For this review, take the finished solid that the model builds, in its own axes (mm). Give positions to 0.01 mm unless a question says otherwise; leave off trailing zeros. Write each loop counter-clockwise with the first axis right and the second up, starting at its lowest first coordinate (ties: lowest second). Pieces come first, ordered by that corner, then holes. Notation, with made-up numbers: (-12, 33.25) -> (44, 33.25) arc R20 ccw to (44, 38.25) -> close; hole circle Ø8 at (79.5, 87). An arc over 180 degrees is marked (long way). Return JSON: item names as keys, results as strings.
from build123d import *

# Parameters (mm, degrees)
F0_R     = 2.75
F1_DEPTH = 6


with BuildPart() as f1:
    # F0 (on Top) → F1 (new body)
    with BuildSketch(Plane.XY):
        with BuildLine():
            Line((6.000003, -2.478286), (-4.999997, -2.478286))
            Line((-4.999997, -2.478286), (-4.999997, -8.478286))
            ThreePointArc((-4.999997, -8.478286), (0.37213, -14.229707), (6.000003, -8.728286))
            Line((6.000003, -8.728286), (6.000003, -2.478286))
        make_face()
        with Locations((0.497162, -8.728286)):
            Circle(F0_R, mode=Mode.SUBTRACT)
    extrude(amount=F1_DEPTH)


solid = f1.part
1. For pin 1 (1.5 mm diameter, centred on x = 0, y = -11, fed in from +Z); pin 2 (3.5 mm diameter, centred on x = 0.5, y = -8.73, fed in from +Z); pin 3 (2 mm diameter, centred on y = -12, z = 1, fed in from -X), all flat-tipped, find the tip position at first contact; note any pin that passes through.
Results found:
{"pin 1": "stops at z = 6", "pin 2": "passes through", "pin 3": "stops at x = -4.51"}
2. To check wall thickness, follow probe 1 along X at (y, z) = (-5.5, 0.85); probe 2 along Y at (x, z) = (1, 1.1); probe 3 along X at (y, z) = (-10.5, 1.3). State the ranges of each line that lie inside material, in increasing order.
Results found:
{"probe 1": "x = -5 to 6", "probe 2": "y = -14.21 to -11.43, -6.02 to -2.48", "probe 3": "x = -4.71 to -1.61, 2.6 to 5.71"}
3. Add section C-C, the plane y = -8. State the section outline as (x, z) points, plus the area to 3 significant figures.
Results found:
{"outline": "(-5, 0) -> (-2.15, 0) -> (-2.15, 6) -> (-5, 6) -> close; (3.15, 0) -> (6, 0) -> (6, 6) -> (3.15, 6) -> close", "area": "34.2 mm²"}
4. Add section A-A, the plane x = 2.5. State the section outline as (y, z) points, plus the area to 3 significant figures.
Results found:
{"outline": "(-13.85, 0) -> (-10.61, 0) -> (-10.61, 6) -> (-13.85, 6) -> close; (-6.84, 0) -> (-2.48, 0) -> (-2.48, 6) -> (-6.84, 6) -> close", "area": "45.6 mm²"}
5. Add section D-D, the plane y = -12.5. State the section outline as (x, z) points, plus the area to 3 significant figures.
Results found:
{"outline": "(-3.51, 0) -> (4.5, 0) -> (4.5, 6) -> (-3.51, 6) -> close", "area": "48.1 mm²"}
6. The part is to be moulded in two halves that separate along X. For faces 1 (the flat face through (0.4, -5.7, 6)), 2 (the flat face through (6, -6, 3)), 3 (the cylindrical face through (0.249, -14.226, 2.958)), 4 (the cylindrical face through (-0.099, -11.413, 2.958)), say which applies: +X half, -X half, draft (parallel to the pull), parting line (faces both ways), or undercut.
Results found:
{"face 1": "draft", "face 2": "+X half", "face 3": "parting line", "face 4": "undercut"}
